from build123d import *

# Parameters (mm, degrees)
F0_W     = 133.553728
F0_H     = 59.615288
F1_DEPTH = 12.7
F2_DEPTH = 11.43
F0_W_2   = 15.333298
F0_H_2   = 8.458886
F3_DEPTH = 10.16
F4_DEPTH = 12.7


with BuildPart() as f1:
    # F0 (on Front) → F1 (new body, symmetric)
    with BuildSketch(Plane.XZ):
        Polygon((71.228367, -33.870557), (71.228367, 33.870557), (-71.228367, 33.870557), (-71.228367, -33.870557), (-7.538104, -33.870557), (7.795194, -33.870557), align=None)
        Rectangle(F0_W, F0_H, mode=Mode.SUBTRACT)
    extrude(amount=F1_DEPTH, both=True)

    # F0 (on Front) → F2 (join, symmetric)
    with BuildSketch(Plane.XZ):
        Rectangle(F0_W, F0_H)
    extrude(amount=F2_DEPTH, both=True)

    # F0 (on Front) → F3 (join, symmetric)
    with BuildSketch(Plane.XZ):
        with Locations((0.128545, -38.1)):
            Rectangle(F0_W_2, F0_H_2)
    extrude(amount=F3_DEPTH, both=True)

    # F0 (on Front) → F4 (join, symmetric)
    with BuildSketch(Plane.XZ):
        Polygon((35.614184, -42.329443), (7.795194, -42.329443), (-7.538104, -42.329443), (-35.614184, -42.329443), (-35.614184, -44.638067), (35.614184, -44.638067), align=None)
    extrude(amount=F4_DEPTH, both=True)


solid = f1.part
Verification items for the finished model (mm, model axes). A direction names the side the tool comes from. Round coordinates to 2 decimals unless told otherwise and drop trailing zeros. Loops run counter-clockwise (first coordinate to the right, second up) from the corner with the lowest first, then second, coordinate; pieces in that order, holes last. Notation, with made-up numbers: (62.25, -12) - (100.25, -12) arc R20 ccw to (100.25, -6) - close; hole circle Ø1 at (-25.5, 43). An arc over 180 degrees is marked (long way). Answer in a Markdown table with one row per item. Add a question column.
Q1. Material ranges on line 1 (Z direction, x = 35, y = 5.5); line 2 (Y direction, x = 8.5, z = -21); line 3 (Z direction, x = 57, y = -3), recorded low to high.
Q2. Section check B-B on y = -5.5. Enter the section's corners in (x, z).
Q3. Section check D-D on z = -38. Enter the section's corners in (x, y), plus the area to 3 significant figures.
Q4. Release check for a two-part mould opening along Z. For faces 1 (the face through (0, 0, -44.638)), 2 (the face through (-6, -12.7, -30)), 3 (the face through (-1, 11.43, 0)) record: pulls with the +Z half, pulls with the -Z half, needs draft (parallel to the pull), parting line crosses it, or undercut.
Q5. Gauge pin test, flat ends, axial feed: pin 1 (0.7 mm diameter, centred on y = 0.5, z = -43, fed in from -X); pin 2 (6 mm diameter, centred on x = 39.5, y = -4.5, fed in from -Z); pin 3 (10 mm diameter, centred on x = 24.5, z = -15.5, fed in from +Y). Record the tip position at first contact, or that the pin passes through.
Q6. Tool access check on faces 4 (the face through (-7.538, 0, -38)), 5 (the face through (0, 10.16, -38)), 6 (the face through (-1, -11.43, 0)), 7 (the face through (7.795, 0, -38)), 8 (the face through (0, -10.16, -38)). Record the directions out of +Z, -Z, +X, -X, +Y, -Y that give a thin tool (end or side, any length) a straight path to the whole face; none if there is none.
Q7. Section check C-C on x = 42. Enter the section's corners in (y, z), plus the area to 3 significant figures.
Q8. Section check A-A on x = -26.5. Enter the section's corners in (y, z), plus the area to 3 significant figures.
Found:
| question | item | result |
|---|---|---|
| 1 | line 1 | z = -44.64 to -42.33, -33.87 to 33.87 |
| 1 | line 2 | y = -11.43 to 11.43 |
| 1 | line 3 | z = -33.87 to 33.87 |
| 2 | outline | (-71.23, -33.87) - (-7.54, -33.87) - (-7.54, -42.33) - (-35.61, -42.33) - (-35.61, -44.64) - (35.61, -44.64) - (35.61, -42.33) - (7.8, -42.33) - (7.8, -33.87) - (71.23, -33.87) - (71.23, 33.87) - (-71.23, 33.87) - close |
| 3 | outline | (-7.54, -10.16) - (7.8, -10.16) - (7.8, 10.16) - (-7.54, 10.16) - close |
| 3 | area | 312 mm² |
| 4 | face 1 | pulls with the -Z half |
| 4 | face 2 | needs draft |
| 4 | face 3 | undercut |
| 5 | pin 1 | stops at x = -35.61 |
| 5 | pin 2 | stops at z = -33.87 |
| 5 | pin 3 | stops at y = 11.43 |
| 6 | face 4 | -X, +Y, -Y |
| 6 | face 5 | +X, -X, +Y |
| 6 | face 6 | -Y |
| 6 | face 7 | +X, +Y, -Y |
| 6 | face 8 | +X, -X, -Y |
| 7 | outline | (-12.7, -33.87) - (12.7, -33.87) - (12.7, -29.81) - (11.43, -29.81) - (11.43, 29.81) - (12.7, 29.81) - (12.7, 33.87) - (-12.7, 33.87) - (-12.7, 29.81) - (-11.43, 29.81) - (-11.43, -29.81) - (-12.7, -29.81) - close |
| 7 | area | 1,570 mm² |
| 8 | outline | (-12.7, -44.64) - (12.7, -44.64) - (12.7, -42.33) - (-12.7, -42.33) - close; (-12.7, -33.87) - (12.7, -33.87) - (12.7, -29.81) - (11.43, -29.81) - (11.43, 29.81) - (12.7, 29.81) - (12.7, 33.87) - (-12.7, 33.87) - (-12.7, 29.81) - (-11.43, 29.81) - (-11.43, -29.81) - (-12.7, -29.81) - close |
| 8 | area | 1,630 mm² |
